```python
from build123d import *

# Parameters (mm, degrees)
SKETCH_W        = 70
SKETCH_H        = 40
PAD_DEPTH       = 4
SKETCH001_W     = 5
SKETCH001_H     = 2
PAD001_DEPTH    = 35
SKETCH002_R     = 1.3
POCKET_DEPTH    = 37
SKETCH003_R     = 1.5
POCKET001_DEPTH = 5


with BuildPart() as part:
    # Sketch → Pad (new body)
    with BuildSketch(Plane.XY):
        with Locations((35, 20)):
            Rectangle(SKETCH_W, SKETCH_H)
    extrude(amount=PAD_DEPTH)

    # Sketch001 (on Face6 of Pad) → Pad001 (join)
    with BuildSketch(Plane.XY.offset(4)):
        with Locations((35, 36.5)):
            Rectangle(SKETCH001_W, SKETCH001_H)
        with Locations((35, 3.5)):
            Rectangle(SKETCH001_W, SKETCH001_H)
    extrude(amount=PAD001_DEPTH)

    # Sketch002 (on Face8 of Pad001) → Pocket (cut)
    with BuildSketch(Plane.XZ.offset(-2.5)):
        with Locations((35, 35)):
            Circle(SKETCH002_R)
    extrude(amount=-POCKET_DEPTH, mode=Mode.SUBTRACT)

    # Sketch003 (on Face4 of Pocket) → Pocket001 (cut)
    with BuildSketch(Plane(origin=(0, 0, 0), x_dir=(1, 0, 0), z_dir=(0, 0, -1))):
        with Locations((18, -20)):
            Circle(SKETCH003_R)
        with Locations((52, -20)):
            Circle(SKETCH003_R)
    extrude(amount=-POCKET001_DEPTH, mode=Mode.SUBTRACT)


solid = part.part
```
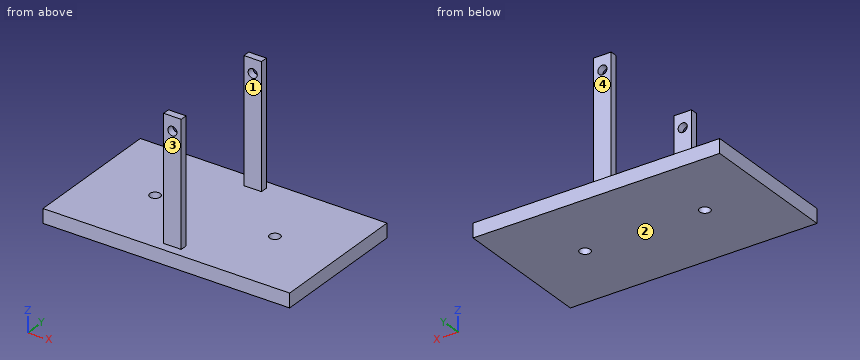
Part model, mm, in its own coordinate system. Face numbers are marked on the shaded views. Round coordinates to 2 decimals unless told otherwise and drop trailing zeros. Loops run counter-clockwise (first coordinate to the right, second up) from the corner with the lowest first, then second, coordinate; pieces in that order, holes last. Notation, with made-up numbers: (-14.5, 45.25) -> (38.5, 45.25) arc R23 ccw to (38.5, 57.25) -> close; hole circle Ø8 at (8, 80.5). An arc over 180 degrees is marked (long way). Use CSV: the item, a comma, the result in double quotes. Start each with the question number.
1) Cut at B-B, the plane x = 18. Write the cut outline in (y, z), plus the area to 3 significant figures.
2) Pull direction Y, two halves, no side cores. Call the marked faces 1, 2, 3 and 4: +Y half, -Y half, draft (parallel to the pull), parting line (faces both ways), or undercut.
3) Wall check: L1, parallel to X at y = 20, z = 1; L2, parallel to Z at x = 35, y = 36.6; L3, parallel to Y at x = 52, z = 3.1. Give the ranges that are in metal, low to high. Write a range as [from, to].
4) Cut at C-C, the plane y = 20. Write the cut outline in (x, z), plus the area to 3 significant figures.
5) Cut at A-A, the plane z = 21. Write the cut outline in (x, y).
6) Drop flat-ended pins along their axis: P1, Ø10, axis at x = 40, y = 22, coming from the +Z side; P2, Ø1.5, axis at x = 34, z = 24, coming from the +Y side; P3, Ø1.6, axis at y = 36.5, z = 25.5, coming from the -X side. Give the stop position or say it passes through.
7) Cut at D-D, the plane z = 35. Write the cut outline in (x, y).
Determined:
1,outline,"(0, 0) -> (18.5, 0) -> (18.5, 4) -> (0, 4) -> close; (21.5, 0) -> (40, 0) -> (40, 4) -> (21.5, 4) -> close"
1,area,"148 mm2"
2,face 1,"undercut"
2,face 2,"draft"
2,face 3,"-Y half"
2,face 4,"+Y half"
3,L1,"x = [0, 16.5], [19.5, 50.5], [53.5, 70]"
3,L2,"z = [0, 33.7], [36.3, 39]"
3,L3,"y = [0, 18.5], [21.5, 40]"
4,outline,"(0, 0) -> (16.5, 0) -> (16.5, 4) -> (0, 4) -> close; (19.5, 0) -> (50.5, 0) -> (50.5, 4) -> (19.5, 4) -> close; (53.5, 0) -> (70, 0) -> (70, 4) -> (53.5, 4) -> close"
4,area,"256 mm2"
5,outline,"(32.5, 2.5) -> (37.5, 2.5) -> (37.5, 4.5) -> (32.5, 4.5) -> close; (32.5, 35.5) -> (37.5, 35.5) -> (37.5, 37.5) -> (32.5, 37.5) -> close"
6,P1,"stops at z = 4"
6,P2,"stops at y = 37.5"
6,P3,"stops at x = 32.5"
7,outline,"(32.5, 2.5) -> (33.7, 2.5) -> (33.7, 4.5) -> (32.5, 4.5) -> close; (32.5, 35.5) -> (33.7, 35.5) -> (33.7, 37.5) -> (32.5, 37.5) -> close; (36.3, 2.5) -> (37.5, 2.5) -> (37.5, 4.5) -> (36.3, 4.5) -> close; (36.3, 35.5) -> (37.5, 35.5) -> (37.5, 37.5) -> (36.3, 37.5) -> close"
